Source: CAD feature listing. Evaluate the final solid. Frame: model axes, mm. Face numbers are marked on the shaded views. A direction names the side the tool comes from. Give positions to 0.01 mm unless a question says otherwise; leave off trailing zeros. Write each loop counter-clockwise with the first axis right and the second up, starting at its lowest first coordinate (ties: lowest second). Pieces come first, ordered by that corner, then holes.
```python
from build123d import *

# Parameters (mm, degrees)
SKETCH2_W           = 323.85
SKETCH2_H           = 185.42
BOSS_EXTRUDE1_DEPTH = 25.4
SKETCH3_W           = 158.75
SKETCH3_H           = 133.35
CUT_EXTRUDE2_DEPTH  = 25.4


with BuildPart() as part:
    # Sketch2 → Boss-Extrude1 (new body)
    with BuildSketch(Plane(origin=(0, 0, 0), x_dir=(1, 0, 0), z_dir=(0, 1, 0))):
        with Locations((8.034446565, -16.382757634)):
            Rectangle(SKETCH2_W, SKETCH2_H)
    extrude(amount=BOSS_EXTRUDE1_DEPTH)

    # Sketch3 → Cut-Extrude2 (cut)
    with BuildSketch(Plane(origin=(0, 25.4, 0), x_dir=(1, 0, 0), z_dir=(0, 1, 0))):
        Polygon((-153.890553435, 24.257242366), (-153.890553435, -12.50606057), (-153.890553435, -109.092757634), (-31.970553435, -109.092757634), (-31.970553435, 24.257242366), align=None)
        with Locations((90.584446565, -42.417757634)):
            Rectangle(SKETCH3_W, SKETCH3_H)
    extrude(amount=-CUT_EXTRUDE2_DEPTH, mode=Mode.SUBTRACT)


solid = part.part
```
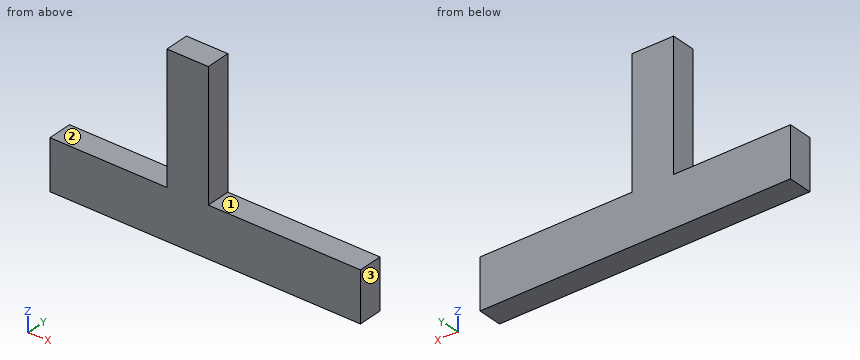
1. Access query for the marked faces 1, 2 and 3. Directions: +Z, -Z, +X, -X, +Y, -Y. A direction counts if a zero-diameter tool reaches every point of the face in a straight line with its end or side. Return the directions, or none.
2. Cut plane B-B, the plane z = -11.5. Return the cut outline in (x, y), then the cut area to 3 significant figures.
3. Contact query for flat-ended pins moving along their axis: P1, Ø12, axis at y = 18, z = -18, coming from the -X side; P2, Ø7.5, axis at x = -99.5, y = 16.5, coming from the +Z side; P3, Ø1.5, axis at x = -29.5, z = 49.5, coming from the -Y side. Output: stop coordinate, or through.
4. Cut plane C-C, the plane x = 105.5. Return the cut outline in (y, z), then the cut area to 3 significant figures.
5. Cut plane A-A, the plane y = 9.5. Return the cut outline in (x, z).
6. Line query: L1, parallel to X at y = 1.75, z = -0.5; L2, parallel to Z at x = 18.5, y = 15. Output: solid intervals per line, ascending.
Response values:
1. face 1: +Z, +X, +Y, -Y
1. face 2: +Z, -X, +Y, -Y
1. face 3: +Z, -Z, +X, +Y, -Y
2. outline: (-31.97, 0) - (11.21, 0) - (11.21, 25.4) - (-31.97, 25.4) - close
2. area: 1,100 mm2
3. P1: stops at x = -31.97
3. P2: stops at z = -24.26
3. P3: stops at y = 0
4. outline: (0, -76.33) - (25.4, -76.33) - (25.4, -24.26) - (0, -24.26) - close
4. area: 1,320 mm2
5. outline: (-153.89, -76.33) - (169.96, -76.33) - (169.96, -24.26) - (11.21, -24.26) - (11.21, 109.09) - (-31.97, 109.09) - (-31.97, -24.26) - (-153.89, -24.26) - close
6. L1: x = -31.97 to 11.21
6. L2: z = -76.33 to -24.26
